from build123d import *

# Parameters (mm, degrees)
F0_R           = 6.35
F1_DEPTH       = 6.35
F2_D           = 3.7973
F2_CSINK_D     = 7.7978
F2_CSINK_ANGLE = 82
F3_C1_SIZE     = 1.5875
F3_C2_SIZE     = 1.5875
F3_C3_SIZE     = 1.5875
F3_C4_SIZE     = 1.5875
F3_C5_SIZE     = 1.5875


with BuildPart() as f1:
    # F0 (on Top) → F1 (new body)
    with BuildSketch(Plane.XY):
        with BuildLine():
            Line((-87.0919269209, -13.7156903623), (-87.0919269209, -14.792130794))
            Line((-87.0919269209, -14.792130794), (106.5325381816, -14.792130794))
            Line((106.5325381816, -14.792130794), (106.5325381816, -14.3110791923))
            ThreePointArc((106.5325381816, -14.3110791923), (106.846778333, -12.3382378278), (107.7583974098, -10.5606550362))
            ThreePointArc((107.7583974098, -10.5606550362), (111.5641860478, 1.082869206), (107.7583974098, 12.7263934482))
            ThreePointArc((107.7583974098, 12.7263934482), (106.846778333, 14.5039762398), (106.5325381816, 16.4768176043))
            Line((106.5325381816, 16.4768176043), (106.5325381816, 16.957869206))
            Line((106.5325381816, 16.957869206), (-87.0919269209, 16.957869206))
            Line((-87.0919269209, 16.957869206), (-87.0919269209, 15.8814287743))
            ThreePointArc((-87.0919269209, 15.8814287743), (-87.3716340972, 14.0175497454), (-88.1861143334, 12.3178723984))
            ThreePointArc((-88.1861143334, 12.3178723984), (-91.6358139522, 1.082869206), (-88.1861143334, -10.1521339864))
            ThreePointArc((-88.1861143334, -10.1521339864), (-87.3716340972, -11.8518113334), (-87.0919269209, -13.7156903623))
        make_face()
        with Locations((-34.4858139522, 1.082869206)):
            Circle(F0_R, mode=Mode.SUBTRACT)
    extrude(amount=-F1_DEPTH)

    # F2 (through all)
    with Locations(Plane.XY):
        with Locations((102.0391860478, 1.082869206), (-82.1108139522, 1.082869206)):
            CounterSinkHole(F2_D / 2, F2_CSINK_D / 2, counter_sink_angle=F2_CSINK_ANGLE)

    # F3: chamfer of 1.5875 on 9 edges, made by hand

    # F3_c1
    f3_c1_edges = [f1.edges().sort_by_distance(p)[0] for p in [
        (-87.3716340972, -11.8518113334, 0),
        (-91.6358139522, 1.082869206, 0),
        (-87.0919269209, -14.2539105781, 0),
        (-87.3716340972, 14.0175497454, 0),
        (-87.0919269209, 16.4196489902, 0),
    ]]
    chamfer(f3_c1_edges, length=F3_C1_SIZE)

    # F3_c2
    f3_c2_edges = [f1.edges().sort_by_distance(p)[0] for p in [
        (-87.3716340972, -11.8518113334, -6.35),
        (-91.6358139522, 1.082869206, -6.35),
        (-87.0919269209, -14.2539105781, -6.35),
        (-87.3716340972, 14.0175497454, -6.35),
        (-87.0919269209, 16.4196489902, -6.35),
    ]]
    chamfer(f3_c2_edges, length=F3_C2_SIZE)

    # F3_c3
    f3_c3_edges = [f1.edges().sort_by_distance(p)[0] for p in [
        (106.5325381816, -14.5516049932, 0),
        (106.846778333, -12.3382378278, 0),
        (106.5325381816, 16.7173434052, 0),
        (111.5641860478, 1.082869206, 0),
        (106.846778333, 14.5039762398, 0),
    ]]
    chamfer(f3_c3_edges, length=F3_C3_SIZE)

    # F3_c4
    f3_c4_edges = [f1.edges().sort_by_distance(p)[0] for p in [
        (9.7203056303, -14.792130794, 0),
    ]]
    chamfer(f3_c4_edges, length=F3_C4_SIZE)

    # F3_c5
    f3_c5_edges = [f1.edges().sort_by_distance(p)[0] for p in [
        (9.7203056303, 16.957869206, 0),
    ]]
    chamfer(f3_c5_edges, length=F3_C5_SIZE)


solid = f1.part
For this review, take the finished solid that the model builds, in its own axes (mm). Coordinates: 2 decimals unless noted, no trailing zeros. Order: outer loops, then holes, each group sorted by start corner. A loop starts at its lowest first (then second) coordinate and runs counter-clockwise, first axis right, second up. Notation, with made-up numbers: (53, -10) - (97, -10) arc R27 ccw to (97, 27) - close; hole circle Ø9 at (61.5, -39). An arc over 180 degrees is marked (long way). Use one line per item in the form item = value.
Q1. Consider section A-A (z = -3.5). Give the boundary of the cut face in (x, y).
Checked values:
outline = (-88.19, -10.15) arc R6.35 cw to (-87.09, -13.72) - (-87.09, -14.79) - (106.53, -14.79) - (106.53, -14.31) arc R6.35 cw to (107.76, -10.56) arc R19.71 ccw to (107.76, 12.73) arc R6.35 cw to (106.53, 16.48) - (106.53, 16.96) - (-87.09, 16.96) - (-87.09, 15.88) arc R6.35 cw to (-88.19, 12.32) arc R20.02 ccw to start; hole circle Ø3.8 at (-82.11, 1.08); hole circle Ø12.7 at (-34.49, 1.08); hole circle Ø3.8 at (102.04, 1.08)
Q2. Draft analysis for pull direction Y (two halves, no side actions). For faces 1 (the cylindrical face through (-80.214, 1.166, -4.354)), 2 (the cylindrical face through (-91.635, 1.25, -3.153)), 3 (the flat face through (8, -14.792, -4)), state which applies: +Y half, -Y half, draft (parallel to the pull), parting line (faces both ways), or undercut.
Checked values:
face_1 = undercut
face_2 = parting line
face_3 = -Y half
Q3. For probe 1 along X at (y, z) = (0.5, -2); probe 2 along X at (y, z) = (-4.5, -3.5); probe 3 along X at (y, z) = (-3.5, -4), list the stretches that pass through material, from the lowest coordinate up. Write a range as from..to.
Checked values:
probe_1 = -91.63..-84.19, -80.03..-40.81, -28.16..99.96, 104.12..111.56
probe_2 = -90.84..-37.51, -31.46..110.76
probe_3 = -91.1..-38.88, -30.09..111.02
Q4. For P1, Ø0.5, axis at y = -14.5, z = -3.5, coming from the +X side; P2, Ø4.5, axis at x = -82.11, y = 1.08, coming from the +Z side; P3, Ø0.5, axis at y = -14.5, z = -3, coming from the -X side; P4, Ø7.5, axis at x = -34.49, y = 1.08, coming from the -Z side, all flat-tipped, find the tip position at first contact; note any pin that passes through.
Checked values:
P1 = 106.53
P2 = -1.89
P3 = -87.09
P4 = through
